Autodesk Inventor part; units mm, degrees
ref_plane "Work Plane1" through (0, 0, 0) normal (0, 0, 1) x (1, 0, 0)
ref_plane "YZ Plane" through (0, 0, 0) normal (1, 0, 0) x (0, 1, 0)
ref_plane "XZ Plane" through (0, 0, 0) normal (0, 1, 0) x (-1, 0, 0)
sketch "Sketch1" plane through (0, 0, 0) normal (0, 1, 0) x (-1, 0, 0)
  line L0 (325, -187.6388) -> (0, -375.2777)
  line L1 (0, -375.2777) -> (-325, -187.6388)
  line L2 (-325, -187.6388) -> (-325, 187.6388)
  line L3 (-325, 187.6388) -> (0, 375.2777)
  line L4 (0, 375.2777) -> (325, 187.6388)
  line L5 (325, 187.6388) -> (325, -187.6388)
  point P0 (0, 0)
  point P1 (0, 0)
  point P2 (325, 0)
extrude "Extrusion1" add sketch "Sketch1" against normal blind 265
sketch "Sketch2" plane through (0, -265, 0) normal (0, -1, 0) x (1, 0, 0)
  circle A0 centre (0, 0) radius 200
  dimension "d4" = 400
extrude "Extrusion2" add sketch "Sketch2" along normal blind 1500
chamfer "Chamfer1" distance 25 angle 45 1 edges at (-200, -1765, 0)
ref_plane "Work Plane1" through (0, 0, 0) normal (0, 0, 1) x (1, 0, 0)
sketch "Sketch3" plane through (0, 0, 0) normal (0, 0, 1) x (1, 0, 0)
  point P0 (0, 0)
sketch "Sketch4" plane through (0, 0, 0) normal (0, 0, 1) x (1, 0, 0)
  line L0 (0, 0) -> (275, 0)
  line L1 (0, 0) -> (325, 0)
  line L2 (275, 0) -> (497.8484, -144.7195)
  line L3 (275, 0) -> (540.7163, 0) construction
  line L4 (497.8484, -144.7195) -> (497.8484, 0)
  line L5 (497.8484, 0) -> (275, 0)
  line L6 (0, -2118) -> (0, 353)
  dimension "d11" = 275
  dimension "d12" = 33
revolve "Revolution1" cut sketch "Sketch4" angle 360 about axis through (0, -10, 0) along (0, 1, 0)
Input: part model. Units: mm. Frame: model coordinates. A direction names the side the tool comes from. Give positions to 0.01 mm unless a question says otherwise; leave off trailing zeros. Write each loop counter-clockwise with the first axis right and the second up, starting at its lowest first coordinate (ties: lowest second). Pieces come first, ordered by that corner, then holes.
Q1. First-contact query: P1, Ø3, axis at y = -1560, z = 88, coming from the +X side; P2, Ø4, axis at y = -783.5, z = -67, coming from the +X side; P3, Ø8, axis at y = -1228, z = -164.5, coming from the -X side. Flat tips, straight axial feed; report the tip coordinate or a pass-through.
Q2. Section B-B, the plane y = -158. Output: boundary loops of the cut face in (x, z).
Q3. Material intervals for probe 1 along Y at (x, z) = (-111, 239.5); probe 2 along X at (y, z) = (-198.5, -340); probe 3 along X at (y, z) = (-1239.5, -130), sorted ascending.
Q4. Section C-C, the plane y = -769. Output: boundary loops of the cut face in (x, z), plus the area to 3 significant figures.
Q5. Section A-A, the plane z = 0. Output: boundary loops of the cut face in (x, y).
Q6. Set-up query: faces 1 (the face through (164.78, -147.11, 280.14)), 2 (the face through (149, -265, -162)). Return all of +Z, -Z, +X, -X, +Y, -Y with unobstructed straight access to the full face (end or side cutting, diameter ignored); none if empty.
Filled in:
1. P1: stops at x = 180.33
1. P2: stops at x = 189.14
1. P3: stops at x = -119.33
2. outline: (-325, -187.64) - (0, -375.28) - (325, -187.64) - (325, 187.64) - (0, 375.28) - (-325, 187.64) - close
3. probe 1: y = -265 to 0
3. probe 2: x = -61.1 to 61.1
3. probe 3: x = -151.99 to 151.99
4. outline: circle Ø400 at (0, 0)
4. area: 126,000 mm2
5. outline: (-325, -265) - (-200, -265) - (-200, -1740) - (-175, -1765) - (175, -1765) - (200, -1740) - (200, -265) - (325, -265) - (325, -32.47) - (275, 0) - (-275, 0) - (-325, -32.47) - close
6. face 1: +Z, +X, +Y, -Y
6. face 2: -Y
